Could you check a few things on this drawing? It's one solid part, dimensions in mm from its lowest x, y, z. A direction names the side the tool comes from. Round coordinates to 2 decimals unless told otherwise and drop trailing zeros. Loops run counter-clockwise (first coordinate to the right, second up) from the corner with the lowest first, then second, coordinate; pieces in that order, holes last. Notation, with made-up numbers: (17, -23.75) -> (65, -23.75) arc R30 ccw to (65, 3.25) -> close; hole circle Ø5 at (5, 80). An arc over 180 degrees is marked (long way). Use CSV: the item, a comma, the result in double quotes. Start each with the question number.
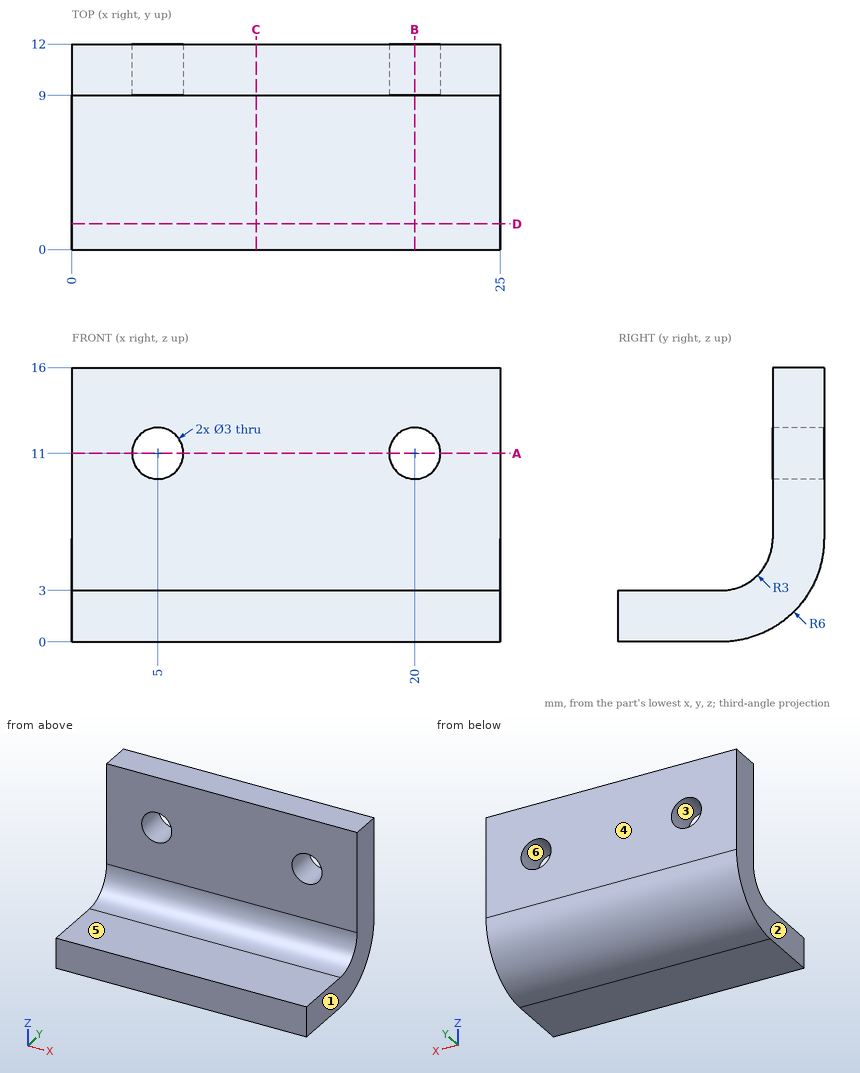
Q1. I want a section at B-B, the plane x = 20. List the corners of the cut face in (y, z) for me.
Q2. I want a section at D-D, the plane y = 1.5. List the corners of the cut face in (x, z) for me, then the cut area to 3 significant figures.
Q3. I want a section at C-C, the plane x = 10.75. List the corners of the cut face in (y, z) for me, then the cut area to 3 significant figures.
Q4. For the marked faces 5 and 6, which set-ups out of +Z, -Z, +X, -X, +Y, -Y let a thin tool reach every point of the face, with its end or its side?
Q5. If we mould it in two halves opening along X, with no side actions, what happens to the marked faces 1, 2, 3 and 4? For each: pulls with the +X half, pulls with the -X half, needs draft (parallel to the pull), parting line crosses it, or undercut.
Q6. I need wall thicknesses on line 1 along X through (y, z) = (10.2, 11); line 2 along Y through (x, z) = (5, 6.5); line 3 along Z through (x, y) = (6, 4.25). Which ranges of each line are inside material? Lowest first, please.
Q7. Will these pins go through, and if not, where does the flat tip stop? pin 1 Ø5 at (x, y) = (7, 1.5) entering from +Z; pin 2 Ø3.5 at (x, z) = (20, 11) entering from -Y.
Q8. I want a section at A-A, the plane z = 11. List the corners of the cut face in (x, y) for me.
Values found:
1,outline,"(0, 0) -> (6, 0) arc R6 ccw to (12, 6) -> (12, 9.5) -> (9, 9.5) -> (9, 6) arc R3 cw to (6, 3) -> (0, 3) -> close; (9, 12.5) -> (12, 12.5) -> (12, 16) -> (9, 16) -> close"
2,outline,"(0, 0) -> (25, 0) -> (25, 3) -> (0, 3) -> close"
2,area,"75.0 mm2"
3,outline,"(0, 0) -> (6, 0) arc R6 ccw to (12, 6) -> (12, 16) -> (9, 16) -> (9, 6) arc R3 cw to (6, 3) -> (0, 3) -> close"
3,area,"69.2 mm2"
4,face 5,"+Z, +X, -X, -Y"
4,face 6,"+Y, -Y"
5,face 1,"pulls with the +X half"
5,face 2,"pulls with the -X half"
5,face 3,"undercut"
5,face 4,"needs draft"
6,line 1,"0 to 3.5, 6.5 to 18.5, 21.5 to 25"
6,line 2,"9 to 12"
6,line 3,"0 to 3"
7,pin 1,"z = 3"
7,pin 2,"y = 9"
8,outline,"(0, 9) -> (3.5, 9) -> (3.5, 12) -> (0, 12) -> close; (6.5, 9) -> (18.5, 9) -> (18.5, 12) -> (6.5, 12) -> close; (21.5, 9) -> (25, 9) -> (25, 12) -> (21.5, 12) -> close"
